from build123d import *


with BuildPart() as f1:
    # F0 (on Right) → F1 (revolve)
    with BuildSketch(Plane.YZ):
        with BuildLine():
            Line((0, 26.166892), (0, 0))
            Line((0, 0), (6.35, 0))
            Line((6.35, 0), (6.35, 3.175))
            ThreePointArc((6.35, 3.175), (5.885032, 4.297532), (4.7625, 4.7625))
            Line((4.7625, 4.7625), (5.007925, 4.7625))
            ThreePointArc((5.007925, 4.7625), (3.425204, 6.226917), (4.7625, 7.918414))
            Line((4.7625, 7.918414), (4.7625, 17.443414))
            ThreePointArc((4.7625, 17.443414), (6.200793, 18.881707), (4.7625, 20.32))
            ThreePointArc((4.7625, 20.32), (3.854894, 24.443781), (0, 26.166892))
        make_face()
    revolve(axis=Axis((0, 0, 13.083446), (0, 0, -1)))


solid = f1.part
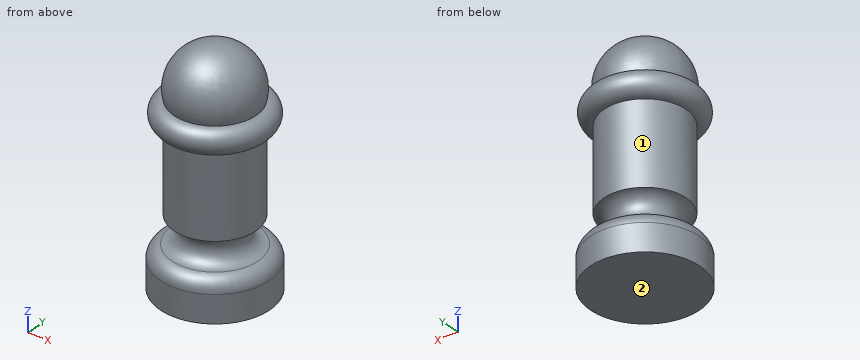
Work out the finished part from the listing and answer in its coordinate system (mm). Face numbers are marked on the shaded views. Give positions to 0.01 mm unless a question says otherwise; leave off trailing zeros. Write each loop counter-clockwise with the first axis right and the second up, starting at its lowest first coordinate (ties: lowest second). Pieces come first, ordered by that corner, then holes. Notation, with made-up numbers: (60, 84) - (96, 84) arc R31 ccw to (96, 109) - close; hole circle Ø11 at (69.5, 67.25). An arc over 180 degrees is marked (long way). One line per item, written item: value. Start each with the question number.
1. Given pin 1 (5 mm diameter, centred on y = 4, z = 13, fed in from +X); pin 2 (1 mm diameter, centred on x = -2, z = 15.5, fed in from -Y); pin 3 (6 mm diameter, centred on x = 0.5, z = 22, fed in from -Y), each flat-ended and moving along its own axis, determine where each tip first touches the part or whether it passes through.
2. Consider probe 1 along Z at (x, y) = (-0.75, 4); probe 2 along Z at (x, y) = (5, -2.75); probe 3 along Z at (x, y) = (3.25, 0.25). Determine where each line is inside the solid, lowest interval first.
3. Find section B-B (z = 6.5). Write down the section's boundary in (x, y), then the cut area to 3 significant figures.
4. For a pull along X with two mould halves and no side action, classify the marked faces 1 and 2 as +X half, -X half, draft (parallel to the pull), parting line (faces both ways), or undercut.
5. Find section A-A (z = 12.5). Write down the section's boundary in (x, y) (1 decimal), then the cut area to 3 significant figures.
Geometry results:
1. pin 1: x = 4.52
1. pin 2: y = -4.52
1. pin 3: y = -6.19
2. probe 1: 0 to 5.07, 7.63 to 24.16
2. probe 2: 0 to 4.45, 17.8 to 19.97
2. probe 3: 0 to 25.05
3. outline: circle Ø6.86 at (0, 0)
3. area: 36.9 mm2
4. face 1: parting line
4. face 2: draft
5. outline: circle Ø9.5 at (0, 0)
5. area: 71.3 mm2
